Verification items for the finished model (mm, model axes). A direction names the side the tool comes from. Round coordinates to 2 decimals unless told otherwise and drop trailing zeros. Order: outer loops, then holes, each group sorted by start corner. A loop starts at its lowest first (then second) coordinate and runs counter-clockwise, first axis right, second up. Notation, with made-up numbers: M 88.5,58.25 L 92.5,58.25 A13 cw 92.5,74.25 Z; hole C 26,54.25 d11. An arc over 180 degrees is marked long. Use CSV: the item, a comma, the result in double quotes. Start each with the question number.
Q1. Sectioned sample at C-C (z = -15). Enter the section's corners in (x, y), and give its area (3 significant figures).
Q2. Gauge pin test, flat ends, axial feed: pin 1 Ø6.5 at (x, y) = (-35.5, 0) entering from -Z; pin 2 Ø6 at (y, z) = (3.5, -31.5) entering from -X; pin 3 Ø6 at (x, z) = (-6, -11) entering from +Y; pin 4 Ø10 at (x, y) = (-22, -16.5) entering from +Z. Record the tip position at first contact, or that the pin passes through.
Q3. Sectioned sample at B-B (y = 0). Enter the section's corners in (x, z).
Q4. Mould release check, pull along X, two halves, no side actions. Record for faces 4 (the face through (-23.675, -4.997, -35.157)), 5 (the face through (-22.19, -13, -2.46)), 6 (the face through (-26.5, 5, -35)), 7 (the face through (-23, 6, -35)): +X half, -X half, draft (parallel to the pull), parting line (faces both ways), or undercut.
Q5. Scan lines: line 1 (Z direction, x = -28, y = -13.5); line 2 (Y direction, x = -23, z = -1); line 3 (Y direction, x = -35.5, z = -2.7). Record each from-to range of solid material in increasing order.
Q6. Sectioned sample at A-A (x = -23.5). Enter the section's corners in (y, z).
Q7. Set-up check for faces 1 (the face through (-12, -2, -5)), 2 (the face through (-20.5, 5, -35)), 3 (the face through (-24, 1, -60)): record each of +Z, -Z, +X, -X, +Y, -Y from which the full face is reachable in a straight line by a thin tool's end or side.
```python
from build123d import *

# Parameters (mm, degrees)
SKETCH8_R           = 22.5
SKETCH8_R_2         = 1.65
BOSS_EXTRUDE5_DEPTH = 10
SKETCH9_R           = 3.65
CUT_EXTRUDE1_DEPTH  = 5
BOSS_EXTRUDE6_DEPTH = 50
FILLET1_R           = 1
CHAMFER1_SIZE       = 2.5


with BuildPart() as part:
    # Sketch8 → Boss-Extrude5 (new body)
    with BuildSketch(Plane(origin=(-41, 0, 0), x_dir=(-1, 0, 0), z_dir=(0, 0, -1))):
        with Locations((-17.5, 0)):
            Circle(SKETCH8_R)
        with Locations((-17.5, 12)):
            Circle(SKETCH8_R_2, mode=Mode.SUBTRACT)
        with Locations((-5.5, 0)):
            Circle(SKETCH8_R_2, mode=Mode.SUBTRACT)
        with Locations((-17.5, -12)):
            Circle(SKETCH8_R_2, mode=Mode.SUBTRACT)
        with Locations((-29.5, 0)):
            Circle(SKETCH8_R_2, mode=Mode.SUBTRACT)
    extrude(amount=BOSS_EXTRUDE5_DEPTH)

    # Sketch9 → Cut-Extrude1 (cut, symmetric)
    with BuildSketch(Plane(origin=(0, 0, -10), x_dir=(-1, 0, 0), z_dir=(0, 0, -1))):
        with Locations((23.5, 12)):
            Circle(SKETCH9_R)
        with Locations((11.5, 0)):
            Circle(SKETCH9_R)
        with Locations((35.5, 0)):
            Circle(SKETCH9_R)
        with Locations((23.5, -12)):
            Circle(SKETCH9_R)
    extrude(amount=CUT_EXTRUDE1_DEPTH, both=True, mode=Mode.SUBTRACT)

    # Sketch10 → Boss-Extrude6 (add)
    with BuildSketch(Plane(origin=(0, 0, -10), x_dir=(-1, 0, 0), z_dir=(0, 0, -1))):
        with BuildLine():
            Line((20.5, 6), (26.5, 6))
            Line((26.5, 6), (26.5, 4))
            ThreePointArc((26.5, 4), (23.5, -5), (20.5, 4))
            Line((20.5, 4), (20.5, 6))
        make_face()
    extrude(amount=BOSS_EXTRUDE6_DEPTH)

    # Fillet1
    fillet1_edges = [part.edges().sort_by_distance(p)[0] for p in [
        (-23.5, -5, -10),
        (-26.5, 5, -10),
        (-23.5, 6, -10),
        (-20.5, 5, -10),
    ]]
    fillet(fillet1_edges, radius=FILLET1_R)

    # Chamfer1
    chamfer1_edges = [part.edges().sort_by_distance(p)[0] for p in [
        (-1, 0, -10),
    ]]
    chamfer(chamfer1_edges, length=CHAMFER1_SIZE)


solid = part.part
```
Verdict:
1,outline,"M -26.5,4 A5 ccw long -20.5,4 L -20.5,6 L -26.5,6 Z"
1,area,"86.5 mm²"
2,pin 1,"stops at z = -5"
2,pin 2,"stops at x = -28.47"
2,pin 3,"stops at y = 14.54"
2,pin 4,"stops at z = 0"
3,outline,"M -46,-7.5 L -43.5,-10 L -39.15,-10 L -39.15,-5 L -37.15,-5 L -37.15,0 L -46,0 Z; M -33.85,-5 L -31.85,-5 L -31.85,-10 L -29.5,-10 A1 cw -28.5,-11 L -28.5,-60 L -18.5,-60 L -18.5,-11 A1 cw -17.5,-10 L -15.15,-10 L -15.15,-5 L -13.15,-5 L -13.15,0 L -33.85,0 Z; M -9.85,-5 L -7.85,-5 L -7.85,-10 L -3.5,-10 L -1,-7.5 L -1,0 L -9.85,0 Z"
4,face 4,"parting line"
4,face 5,"undercut"
4,face 6,"-X half"
4,face 7,"draft"
5,line 1,"z = -10 to 0"
5,line 2,"y = -22.49 to -13.57, -10.43 to 10.43, 13.57 to 22.49"
5,line 3,"y = -19.03 to -1.65, 1.65 to 19.03"
6,outline,"M -22.5,-7.5 L -20,-10 L -15.65,-10 L -15.65,-5 L -13.65,-5 L -13.65,0 L -22.5,0 Z; M -10.35,-5 L -8.35,-5 L -8.35,-10 L -6,-10 A1 cw -5,-11 L -5,-60 L 6,-60 L 6,-11 A1 cw 7,-10 L 8.35,-10 L 8.35,-5 L 10.35,-5 L 10.35,0 L -10.35,0 Z; M 13.65,-5 L 15.65,-5 L 15.65,-10 L 20,-10 L 22.5,-7.5 L 22.5,0 L 13.65,0 Z"
7,face 1,"-Z"
7,face 2,"-Z, +X, +Y"
7,face 3,"-Z, +X, -X, +Y, -Y"
